from build123d import *

# Parameters (mm, degrees)
SKETCH_R      = 1.25
PAD_DEPTH     = 1.5
SKETCH001_R   = 4
PAD001_DEPTH  = 15
SKETCH002_W   = 14.327426
SKETCH002_H   = 14.462592
PAD002_DEPTH  = 1
SKETCH003_R   = 2.5
PAD003_DEPTH  = 9
SKETCH004_W   = 10
SKETCH004_H   = 4.51462
SKETCH004_W_2 = 9.5
SKETCH004_H_2 = 4.078131
SKETCH004_W_3 = 16.5
SKETCH004_H_3 = 3
PAD004_DEPTH  = 5
SKETCH005_W   = 25.572927
SKETCH005_H   = 16.2
PAD005_DEPTH  = 2
SKETCH006_W   = 4.984948
SKETCH006_H   = 9
PAD006_DEPTH  = 5


with BuildPart() as part:
    # Sketch → Pad (new body)
    with BuildSketch(Plane.XY):
        with BuildLine():
            ThreePointArc((-31.5, 35), (-32.56066, 34.56066), (-33, 33.5))
            Line((-33, -33.5), (-33, 33.5))
            ThreePointArc((-33, -33.5), (-32.56066, -34.56066), (-31.5, -35))
            Line((31.5, -35), (-31.5, -35))
            ThreePointArc((31.5, -35), (32.56066, -34.56066), (33, -33.5))
            Line((33, 33.5), (33, -33.5))
            ThreePointArc((33, 33.5), (32.56066, 34.56066), (31.5, 35))
            Line((-31.5, 35), (31.5, 35))
        make_face()
        with Locations((27.75, 29.75)):
            Circle(SKETCH_R, mode=Mode.SUBTRACT)
        with Locations((-27.75, -29.75)):
            Circle(SKETCH_R, mode=Mode.SUBTRACT)
        with Locations((27.75, -29.75)):
            Circle(SKETCH_R, mode=Mode.SUBTRACT)
    extrude(amount=PAD_DEPTH)

    # Sketch001 → Pad001 (join)
    with BuildSketch(Plane.XY):
        with Locations((-28.04706, -5.627252)):
            Circle(SKETCH001_R)
        with Locations((-28.04706, -20.567915)):
            Circle(SKETCH001_R)
    extrude(amount=PAD001_DEPTH)

    # Sketch002 (on DatumPlane) → Pad002 (join)
    with BuildSketch(Plane.XY.offset(1.5)):
        with Locations((-11.592608, 16.860297)):
            Rectangle(SKETCH002_W, SKETCH002_H)
    extrude(amount=PAD002_DEPTH)

    # Sketch003 (on DatumPlane) → Pad003 (join)
    with BuildSketch(Plane.XY.offset(1.5)):
        with Locations((-17.169403, 5.115318)):
            Circle(SKETCH003_R)
        with Locations((-17.169403, -10.668831)):
            Circle(SKETCH003_R)
        with Locations((-11.212177, -10.668831)):
            Circle(SKETCH003_R)
        with Locations((-5.171722, -10.668831)):
            Circle(SKETCH003_R)
    extrude(amount=PAD003_DEPTH)

    # Sketch004 (on DatumPlane) → Pad004 (join)
    with BuildSketch(Plane.XY.offset(1.5)):
        with Locations((-13.5, -30.268985)):
            Rectangle(SKETCH004_W, SKETCH004_H)
        with Locations((-0.789347, -32.460935)):
            Rectangle(SKETCH004_W_2, SKETCH004_H_2)
        with Locations((14.25, -30.987146)):
            Rectangle(SKETCH004_W_3, SKETCH004_H_3)
    extrude(amount=PAD004_DEPTH)

    # Sketch005 (on Face5 of Pad004) → Pad005 (join)
    with BuildSketch(Plane.XY.offset(1.5)):
        with Locations((20.213537, 17.9)):
            Rectangle(SKETCH005_W, SKETCH005_H)
    extrude(amount=PAD005_DEPTH)

    # Sketch006 (on DatumPlane) → Pad006 (join)
    with BuildSketch(Plane.XY.offset(1.5)):
        with Locations((28.390791, -20.5)):
            Rectangle(SKETCH006_W, SKETCH006_H)
    extrude(amount=PAD006_DEPTH)


solid = part.part
The listing builds one solid part. Answer for the finished solid, in the listing's coordinates (mm). A direction names the side the tool comes from. Round coordinates to 2 decimals unless told otherwise and drop trailing zeros. Order: outer loops, then holes, each group sorted by start corner. A loop starts at its lowest first (then second) coordinate and runs counter-clockwise, first axis right, second up. Notation, with made-up numbers: (-31.5, 83) -> (16.5, 83) arc R24 cw to (16.5, 105) -> close; hole circle Ø6 at (-38.75, 57.5). An arc over 180 degrees is marked (long way). Write each question's results on one line, items separated by ' | '. Start each with the question number.
Q1. Find section B-B (y = 29.75). Determine the outline of the cut face in (x, z), then the cut area to 4 significant figures.
Q2. Find section C-C (x = 11). Determine the outline of the cut face in (y, z), then the cut area to 3 significant figures.
Q3. The mould has two halves that part along Y. Classify faces 6 (the cylindrical face through (28.905, 29.271, 0.74)), 7 (the flat face through (-5.539, -32, 4)), 8 (the flat face through (0, 35, 1)): pulls with the +Y half, pulls with the -Y half, needs draft (parallel to the pull), parting line crosses it, or undercut.
Q4. Each of these flat-tipped pins is pushed along its axis until it touches: pin 1 (4 mm diameter, centred on y = -19.5, z = 4, fed in from -X); pin 2 (6 mm diameter, centred on x = -9, y = 6.5, fed in from -Z); pin 3 (3 mm diameter, centred on x = 27.75, y = -29.75, fed in from +Z); pin 4 (1.6 mm diameter, centred on x = 18.5, z = 2.5, fed in from -Y). Where does it stop, or does it pass through?
Q5. Find section A-A (x = 27.75). Determine the outline of the cut face in (y, z).
Q6. Straight lines are drawn through the part: probe 1 along Y at (x, z) = (27.75, 0.75); probe 2 along Y at (x, z) = (18.5, 2.75); probe 3 along Y at (x, z) = (-27.75, 0.85). For each, find the intervals that lie inside material, in ascending order. Write a range as from..to.
Q7. Which of the six approach directions +Z, -Z, +X, -X, +Y, -Y give full straight-line access (tool end or side, diameter ignored) to faces 1 (the flat face through (25.898, -21, 4)), 2 (the cylindrical face through (-19.012, -8.979, 5.937)), 3 (the flat face through (-11, -11, 10.5)), 4 (the flat face through (-1, -32, 6.5)), 5 (the flat face through (28, -16, 4))?
Q8. Find section D-D (z = 5.5). Give the number of separate pieces and of enclosed holes in the cut face, then the cut area to 3 significant figures.
Worked answers:
1) outline: (-33, 0) -> (26.5, 0) -> (26.5, 1.5) -> (-33, 1.5) -> close; (29, 0) -> (33, 0) -> (33, 1.5) -> (29, 1.5) -> close | area: 95.25 mm2
2) outline: (-35, 0) -> (35, 0) -> (35, 1.5) -> (26, 1.5) -> (26, 3.5) -> (9.8, 3.5) -> (9.8, 1.5) -> (-29.49, 1.5) -> (-29.49, 6.5) -> (-32.49, 6.5) -> (-32.49, 1.5) -> (-35, 1.5) -> close | area: 152 mm2
3) face 6: undercut | face 7: needs draft | face 8: pulls with the +Y half
4) pin 1: stops at x = -32.05 | pin 2: stops at z = 0 | pin 3: stops at z = 1.5 | pin 4: stops at y = -32.49
5) outline: (-35, 0) -> (-31, 0) -> (-31, 1.5) -> (-35, 1.5) -> close; (-28.5, 0) -> (28.5, 0) -> (28.5, 1.5) -> (26, 1.5) -> (26, 3.5) -> (9.8, 3.5) -> (9.8, 1.5) -> (-16, 1.5) -> (-16, 6.5) -> (-25, 6.5) -> (-25, 1.5) -> (-28.5, 1.5) -> close; (31, 0) -> (35, 0) -> (35, 1.5) -> (31, 1.5) -> close
6) probe 1: y = -35..-31, -28.5..28.5, 31..35 | probe 2: y = -32.49..-29.49, 9.8..26 | probe 3: y = -35..-31, -28.5..35
7) face 1: +Z, -Y | face 2: +Z | face 3: +Z, +X, +Y, -Y | face 4: +Z, +X, -X, -Y | face 5: +Z, +X, -X
8) separate pieces: 10 | enclosed holes: 0 | area: 357 mm2
